```python
from build123d import *

# Parameters (mm, degrees)
SKETCH_1_R          = 2.5
EXTRUDE_1_DEPTH     = 7
FILLET_1_R          = 1
FILLET_2_R          = 1
FILLET_3_R          = 1
FILLET_4_R          = 1
FILLET_5_R          = 10
SKETCH_2_R          = 7.1
CUT_EXTRUDE_1_DEPTH = 1.6
SKETCH_3_R          = 6.1
CUT_EXTRUDE_2_DEPTH = 4
SKETCH_4_R          = 6.1
CUT_EXTRUDE_4_DEPTH = 4
SKETCH_5_R          = 7.1
CUT_EXTRUDE_5_DEPTH = 1.6
SKETCH_6_R          = 3.5
CUT_EXTRUDE_6_DEPTH = 5
CHAMFER_1_SIZE      = 0.6
CHAMFER_2_SIZE      = 0.5


with BuildPart() as part:
    # 草图1 → 凸台-拉伸1 (new body)
    with BuildSketch(Plane(origin=(0, 0, 0), x_dir=(1, 0, 0), z_dir=(0, 1, 0))):
        with BuildLine():
            Line((-120, 10), (-11.180339887, 10))
            ThreePointArc((-11.180339887, 10), (15, 0), (-11.180339887, -10))
            Line((-11.180339887, -10), (-120, -10))
            ThreePointArc((-120, -10), (-130, 0), (-120, 10))
        make_face()
        with Locations(Location((-11, 0, 0), (0, 0, 270))):
            Circle(SKETCH_1_R, mode=Mode.SUBTRACT)
        with Locations(Location((0, 11, 0), (0, 0, 270))):
            Circle(SKETCH_1_R, mode=Mode.SUBTRACT)
        with Locations(Location((11, 0, 0), (0, 0, 270))):
            Circle(SKETCH_1_R, mode=Mode.SUBTRACT)
        with Locations(Location((0, -11, 0), (0, 0, 270))):
            Circle(SKETCH_1_R, mode=Mode.SUBTRACT)
        Polygon((-104.558275962, -5), (-53.32280907, -5), (-78.940542516, 2.906902245), align=None, mode=Mode.SUBTRACT)
        with BuildLine():
            Line((-111.339745962, 5), (-85.722012516, 5))
            Line((-85.722012516, 5), (-110.343778499, -2.599497322))
            ThreePointArc((-110.343778499, -2.599497322), (-110.084789012, 1.299457992), (-111.339745962, 5))
        make_face(mode=Mode.SUBTRACT)
        Polygon((-72.159072516, 5), (-46.54133907, -2.906902245), (-20.923605624, 5), align=None, mode=Mode.SUBTRACT)
        with BuildLine():
            Line((-39.75986907, -5), (-14.751545054, 2.71880829))
            ThreePointArc((-14.751545054, 2.71880829), (-14.953467696, -1.180594709), (-14.142135624, -5))
            Line((-14.142135624, -5), (-39.75986907, -5))
        make_face(mode=Mode.SUBTRACT)
    extrude(amount=EXTRUDE_1_DEPTH)

    # 圆角1
    fillet_1_edges = [part.edges().sort_by_distance(p)[0] for p in [
        (-85.722012516, 3.5, -5),
        (-111.339745962, 3.5, -5),
        (-110.343778499, 3.5, 2.599497322),
    ]]
    fillet(fillet_1_edges, radius=FILLET_1_R)

    # 圆角2
    fillet_2_edges = [part.edges().sort_by_distance(p)[0] for p in [
        (-104.558275962, 3.5, 5),
        (-53.32280907, 3.5, 5),
        (-78.940542516, 3.5, -2.906902245),
    ]]
    fillet(fillet_2_edges, radius=FILLET_2_R)

    # 圆角3
    fillet_3_edges = [part.edges().sort_by_distance(p)[0] for p in [
        (-46.54133907, 3.5, 2.906902245),
        (-20.923605624, 3.5, -5),
        (-72.159072516, 3.5, -5),
    ]]
    fillet(fillet_3_edges, radius=FILLET_3_R)

    # 圆角4
    fillet_4_edges = [part.edges().sort_by_distance(p)[0] for p in [
        (-39.75986907, 3.5, 5),
        (-14.142135624, 3.5, 5),
        (-14.751545054, 3.5, -2.71880829),
    ]]
    fillet(fillet_4_edges, radius=FILLET_4_R)

    # 圆角5
    fillet_5_edges = [part.edges().sort_by_distance(p)[0] for p in [
        (-11.180339887, 3.5, -10),
        (-11.180339887, 3.5, 10),
    ]]
    fillet(fillet_5_edges, radius=FILLET_5_R)

    # 草图2 → 切除-拉伸1 (cut)
    with BuildSketch(Plane(origin=(0, 0, 0), x_dir=(-1, 0, 0), z_dir=(0, -1, 0))):
        with Locations(Location((0, 0, 0), (0, 0, 90))):
            Circle(SKETCH_2_R)
    extrude(amount=-CUT_EXTRUDE_1_DEPTH, mode=Mode.SUBTRACT)

    # 草图3 → 切除-拉伸2 (cut)
    with BuildSketch(Plane(origin=(0, 0, 0), x_dir=(-1, 0, 0), z_dir=(0, -1, 0))):
        with Locations(Location((120, 0, 0), (0, 0, 90))):
            Circle(SKETCH_3_R)
    extrude(amount=-CUT_EXTRUDE_2_DEPTH, mode=Mode.SUBTRACT)

    # 草图4 → 切除-拉伸4 (cut)
    with BuildSketch(Plane(origin=(0, 7, 0), x_dir=(1, 0, 0), z_dir=(0, 1, 0))):
        with Locations(Location((0, 0, 0), (0, 0, 270))):
            Circle(SKETCH_4_R)
    extrude(amount=-CUT_EXTRUDE_4_DEPTH, mode=Mode.SUBTRACT)

    # 草图5 → 切除-拉伸5 (cut)
    with BuildSketch(Plane(origin=(0, 7, 0), x_dir=(1, 0, 0), z_dir=(0, 1, 0))):
        with Locations(Location((-120, 0, 0), (0, 0, 270))):
            Circle(SKETCH_5_R)
    extrude(amount=-CUT_EXTRUDE_5_DEPTH, mode=Mode.SUBTRACT)

    # 草图6 → 切除-拉伸6 (cut, symmetric)
    with BuildSketch(Plane(origin=(0, 3, 0), x_dir=(1, 0, 0), z_dir=(0, 1, 0))):
        with Locations(Location((0, 0, 0), (0, 0, 270))):
            Circle(SKETCH_6_R)
        with Locations(Location((-120, 0, 0), (0, 0, 270))):
            Circle(SKETCH_6_R)
    extrude(amount=CUT_EXTRUDE_6_DEPTH, both=True, mode=Mode.SUBTRACT)

    # 倒角1
    chamfer_1_edges = [part.edges().sort_by_distance(p)[0] for p in [
        (15, 0, 0),
        (15, 7, 0),
        (-11.83772234, 0, 10.513167019),
        (-11.83772234, 7, 10.513167019),
        (-11.83772234, 0, -10.513167019),
        (-11.83772234, 7, -10.513167019),
        (-130, 0, 0),
        (-67.5, 0, -10),
        (-67.5, 0, 10),
        (-67.5, 7, 10),
        (-67.5, 7, -10),
        (-130, 7, 0),
    ]]
    chamfer(chamfer_1_edges, length=CHAMFER_1_SIZE)

    # 倒角2
    chamfer_2_edges = [part.edges().sort_by_distance(p)[0] for p in [
        (-120, 0, 6.1),
        (0, 7, -6.1),
    ]]
    chamfer(chamfer_2_edges, length=CHAMFER_2_SIZE)


solid = part.part
```
Part model, mm, in its own coordinate system. A direction names the side the tool comes from. Round coordinates to 2 decimals unless told otherwise and drop trailing zeros. Write each loop counter-clockwise with the first axis right and the second up, starting at its lowest first coordinate (ties: lowest second). Pieces come first, ordered by that corner, then holes. Notation, with made-up numbers: M 73,86.25 L 111,86.25 A12 cw 111,99.25 Z; hole C -12,64 d5. An arc over 180 degrees is marked long. One line per question, with ' | ' between items.
(1) 3-axis set-ups, long thin cutter, end or side, ignore diameter. For faces 5 (the face through (-129.6, 6.8, 0.2)), 6 (the face through (-118.3, 5.4, -3.3)), 7 (the face through (-69.019, 3.451, 0.155)): which of +Z, -Z, +X, -X, +Y, -Y reach the whole face in a straight line?
Answer key:
face 5: -X, +Y | face 6: +Y | face 7: +Y, -Y
(2) Pin check, flat tips, straight feed: pin 1 (3.5 mm diameter, centred on x = -46.5, y = 2.5, fed in from +Z); pin 2 (3.5 mm diameter, centred on x = 1.5, z = 2, fed in from +Y); pin 3 (3 mm diameter, centred on y = 1.5, z = 2.5, fed in from +X). Stop position of each tip, or through.
Answer key:
pin 1: stops at z = 10 | pin 2: stops at y = 3 | pin 3: stops at x = 14.97
(3) Probe line 1 along Z through (x, y) = (-117.5, 2); line 2 along X through (y, z) = (5, -11); line 3 along Y through (x, z) = (2.5, 5.5). List the from-to ranges inside material, lowest first.
Answer key:
line 1: z = -10 to -5.56, 5.56 to 10 | line 2: x = -10.64 to -2.5, 2.5 to 10.2 | line 3: y = 1.6 to 3
(4) Saw through at B-B on x = -88. Write the cut outline in (y, z), then the cut area to 3 significant figures.
Answer key:
outline: M 0,-9.4 L 0.6,-10 L 6.4,-10 L 7,-9.4 L 7,-0.11 L 0,-0.11 Z; M 0,5 L 7,5 L 7,9.4 L 6.4,10 L 0.6,10 L 0,9.4 Z | area: 104 mm^2
(5) Saw through at A-A on x = -48.5. Write the cut outline in (y, z).
Answer key:
outline: M 0,-9.4 L 0.6,-10 L 6.4,-10 L 7,-9.4 L 7,-5 L 0,-5 Z; M 0,2.3 L 7,2.3 L 7,9.4 L 6.4,10 L 0.6,10 L 0,9.4 Z
(6) Two-plate mould, pull along X, no slides. Class faces 1 (the face through (-67, 3, 10)), 2 (the face through (-110.084, 3.451, -1.297)), 3 (the face through (-46, 3, -5)), 4 (the face through (-129.6, 0.2, 0.2)): released by +X, released by -X, zero draft, split by the parting line, or undercut.
Answer key:
face 1: zero draft | face 2: undercut | face 3: undercut | face 4: released by -X
